The listing builds one solid part. Answer for the finished solid, in the listing's coordinates (mm). Coordinates: 2 decimals unless noted, no trailing zeros. Order: outer loops, then holes, each group sorted by start corner. A loop starts at its lowest first (then second) coordinate and runs counter-clockwise, first axis right, second up. Notation, with made-up numbers: (-22, 53.25) -> (19, 53.25) arc R12 ccw to (19, 57.25) -> close; hole circle Ø8 at (71, 16.25). An arc over 180 degrees is marked (long way). Answer in a Markdown table with one row per item. Add a question column.
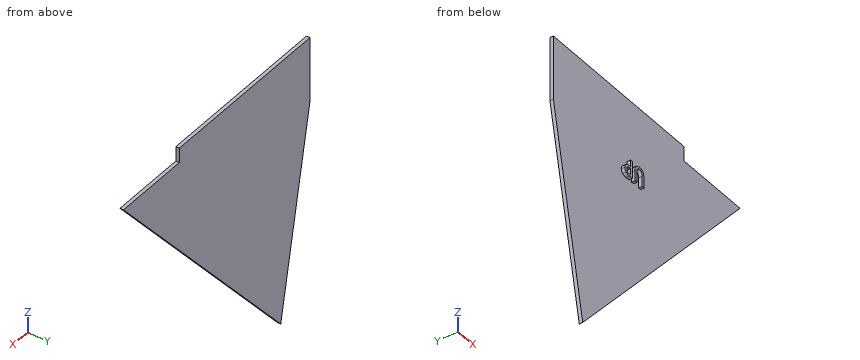
```python
from build123d import *

# Parameters (mm, degrees)
EXTRUDE_1_DEPTH = 1
EXTRUDE_2_DEPTH = 1


with BuildPart() as part:
    # 草图1 → 凸台-拉伸1 (new body)
    with BuildSketch(Plane(origin=(0, 0, 0), x_dir=(1, 0, 0), z_dir=(0, 1, 0))):
        Polygon((12.66597943, 73.92266442), (1, 15.376339461), (1, -3.25), (53, -3.25), (53, 1), (75.227111726, 1), align=None)
    extrude(amount=EXTRUDE_1_DEPTH)

    # 草图2 → 凸台-拉伸2 (add)
    # profile 1 of 2: a face of its own
    with BuildSketch(Plane(origin=(0, 0, 0), x_dir=(1, 0, 0), z_dir=(0, 1, 0))):
        with BuildLine():
            Line((31.090740008, 15.394221889), (30.323543176, 15.394221889))
            Line((30.323543176, 15.394221889), (30.323543176, 17.352620355))
            add(Edge.make_bspline(
                [(30.323543176, 17.352620355), (30.291480188, 17.346927632), (30.225432017, 17.335200902), (30.122464474, 17.325658206), (30.013401991, 17.319675849), (29.938694803, 17.319783871), (29.900262675, 17.319839442)],
                knots=[0, 0, 0, 0, 0.918585764, 1.892241272, 2.915691322, 4, 4, 4, 4], degree=3))
            add(Edge.make_bspline(
                [(29.900262675, 17.319839442), (29.841962947, 17.319869767), (29.726722993, 17.319929711), (29.556261285, 17.335932691), (29.390055361, 17.361937179), (29.228423578, 17.400915644), (29.070924954, 17.451283461), (28.917434146, 17.512464376), (28.768763104, 17.586671732), (28.62561681, 17.671704257), (28.490911455, 17.769835394), (28.373499458, 17.887220571), (28.271718538, 18.019975809), (28.188806413, 18.170044776), (28.12115622, 18.335792286), (28.072018776, 18.517995324), (28.038306105, 18.716089526), (28.030646768, 18.853776873), (28.026679563, 18.925092951)],
                knots=[0, 0, 0, 0, 1.003522523, 1.98364375, 2.944869411, 3.898614004, 4.843729631, 5.790462383, 6.741287792, 7.702146141, 8.655643954, 9.602935836, 10.551034771, 11.527201242, 12.5464735, 13.626777097, 14.770773406, 16, 16, 16, 16], degree=3))
            add(Edge.make_bspline(
                [(28.026679563, 18.925092951), (28.029126999, 18.981235603), (28.033891792, 19.09053695), (28.057781565, 19.249075834), (28.094861108, 19.397722477), (28.143989367, 19.537154386), (28.209760487, 19.66561534), (28.285926292, 19.785665607), (28.377011339, 19.895385017), (28.447566531, 19.958919299), (28.483028853, 19.990852784)],
                knots=[0, 0, 0, 0, 1.126595518, 2.193312949, 3.209115705, 4.196248007, 5.151139266, 6.097382339, 7.043709754, 8, 8, 8, 8], degree=3))
            add(Edge.make_bspline(
                [(28.483028853, 19.990852784), (28.522929015, 20.023049122), (28.603984669, 20.088454754), (28.741989665, 20.169383539), (28.893542525, 20.238034743), (29.059185588, 20.295093718), (29.239564674, 20.338290061), (29.434352813, 20.367230207), (29.64317297, 20.387190847), (29.787147929, 20.388758207), (29.861524951, 20.3895679)],
                knots=[0, 0, 0, 0, 0.838628006, 1.70364077, 2.610636308, 3.559859354, 4.568055018, 5.643200099, 6.782484425, 8, 8, 8, 8], degree=3))
            add(Edge.make_bspline(
                [(29.861524951, 20.3895679), (29.924201068, 20.388442465), (30.046421709, 20.386247828), (30.224716607, 20.380809359), (30.393254737, 20.372443419), (30.551968816, 20.360836156), (30.701043327, 20.348103258), (30.840301091, 20.33201309), (30.969478734, 20.313349379), (31.052038447, 20.298457491), (31.091683908, 20.291306355)],
                knots=[0, 0, 0, 0, 1.217605855, 2.374374404, 3.464660226, 4.494999595, 5.465333604, 6.370582827, 7.217548217, 8, 8, 8, 8], degree=3))
            Line((31.091683908, 20.291306355), (31.090740008, 15.394221889))
        make_face()
        with BuildLine():
            add(Edge.make_bspline(
                [(30.323543176, 19.750609507), (30.294001104, 19.756441871), (30.227115227, 19.76964686), (30.11276139, 19.781736761), (29.973146382, 19.790998313), (29.871306917, 19.79377259), (29.816173468, 19.795274517)],
                knots=[0, 0, 0, 0, 0.708180311, 1.603383121, 2.702528978, 4, 4, 4, 4], degree=3))
            add(Edge.make_bspline(
                [(29.816173468, 19.795274517), (29.778674753, 19.794489016), (29.705419893, 19.792954518), (29.598288212, 19.782736487), (29.496988537, 19.764581207), (29.401019543, 19.740409824), (29.311269908, 19.708215699), (29.227058284, 19.669148461), (29.148784868, 19.623070355), (29.076655109, 19.569835898), (29.010798742, 19.510512464), (28.953667436, 19.442775826), (28.905730333, 19.367849012), (28.86536387, 19.286573026), (28.83427513, 19.198006126), (28.811939273, 19.102330333), (28.797510474, 18.999843052), (28.79510899, 18.929236118), (28.793875472, 18.892968984)],
                knots=[0, 0, 0, 0, 1.164286524, 2.274468469, 3.33712435, 4.356941393, 5.343590938, 6.292901648, 7.23538906, 8.158502959, 9.072142365, 9.981112688, 10.900594105, 11.827687296, 12.792632354, 13.80775062, 14.873954761, 16, 16, 16, 16], degree=3))
            add(Edge.make_bspline(
                [(28.793875472, 18.892968984), (28.795134881, 18.854191832), (28.797580351, 18.778895935), (28.811554204, 18.669650618), (28.835574304, 18.567590725), (28.867328792, 18.472146789), (28.907923347, 18.383372416), (28.95859169, 18.302223365), (29.018603775, 18.228366562), (29.086740761, 18.16077878), (29.163691225, 18.101659974), (29.247154269, 18.048964292), (29.338736059, 18.005658508), (29.437186031, 17.969976467), (29.54264825, 17.941254338), (29.655625397, 17.922037488), (29.775583455, 17.909511306), (29.858027897, 17.907569166), (29.900262675, 17.906574244)],
                knots=[0, 0, 0, 0, 1.10647952, 2.148516939, 3.135813804, 4.093347323, 5.013956832, 5.913991464, 6.814877829, 7.723438285, 8.645449828, 9.577866136, 10.534345172, 11.529217628, 12.562346088, 13.648092354, 14.795160789, 16, 16, 16, 16], degree=3))
            add(Edge.make_bspline(
                [(29.900262675, 17.906574244), (29.941533493, 17.906028809), (30.020359402, 17.904987046), (30.132306289, 17.911998092), (30.23270458, 17.922996362), (30.294355499, 17.937500422), (30.323543176, 17.944367146)],
                knots=[0, 0, 0, 0, 1.161518353, 2.218461969, 3.156558288, 4, 4, 4, 4], degree=3))
            Line((30.323543176, 17.944367146), (30.323543176, 19.750609507))
        make_face(mode=Mode.SUBTRACT)
    # profile 2 of 2: a face of its own
    with BuildSketch(Plane(origin=(0, 0, 0), x_dir=(1, 0, 0), z_dir=(0, 1, 0))):
        with BuildLine():
            Line((32.077134748, 20.358527157), (32.844331579, 20.358527157))
            Line((32.844331579, 20.358527157), (32.844331579, 17.334805283))
            add(Edge.make_bspline(
                [(32.844331579, 17.334805283), (32.846041524, 17.274995945), (32.849340681, 17.159600138), (32.862116571, 16.992717533), (32.883577596, 16.838338831), (32.913517977, 16.696138778), (32.951987807, 16.566089797), (32.999008574, 16.448639235), (33.054117718, 16.34331339), (33.117299737, 16.250152646), (33.189122104, 16.169354435), (33.266600201, 16.098618835), (33.351533105, 16.040070587), (33.442049228, 15.99081552), (33.539783431, 15.954258392), (33.643837974, 15.928897808), (33.754040259, 15.91342912), (33.829727782, 15.911895168), (33.868517376, 15.911109023)],
                knots=[0, 0, 0, 0, 1.442558911, 2.783265207, 4.033293762, 5.19797452, 6.283894868, 7.299176403, 8.243481286, 9.144954945, 10.005756174, 10.844503658, 11.66816234, 12.486940923, 13.323278702, 14.176003432, 15.065208066, 16, 16, 16, 16], degree=3))
            add(Edge.make_bspline(
                [(33.868517376, 15.911109023), (33.904473646, 15.911526383), (33.97484436, 15.912343207), (34.077658287, 15.92781335), (34.174878032, 15.954543092), (34.267116792, 15.991646317), (34.354322253, 16.038718034), (34.435688698, 16.097382655), (34.511493017, 16.167040691), (34.582608735, 16.247198802), (34.646508679, 16.340053843), (34.701762221, 16.445170296), (34.749598601, 16.562786913), (34.787162737, 16.693178193), (34.818776759, 16.835728654), (34.84076289, 16.990817804), (34.855116558, 17.158326046), (34.857473172, 17.274141756), (34.858691406, 17.33401178)],
                knots=[0, 0, 0, 0, 0.880869997, 1.723967724, 2.54076827, 3.348096003, 4.15667844, 4.964596865, 5.80091263, 6.676282017, 7.586647838, 8.557371955, 9.582678263, 10.694376867, 11.880403812, 13.160330013, 14.532054847, 16, 16, 16, 16], degree=3))
            Line((34.858691406, 17.33401178), (34.858691406, 20.358527157))
            Line((34.858691406, 20.358527157), (35.625888237, 20.358527157))
            Line((35.625888237, 20.358527157), (35.625888237, 17.380520301))
            add(Edge.make_bspline(
                [(35.625888237, 17.380520301), (35.623936714, 17.291573771), (35.620165761, 17.119701207), (35.595302232, 16.872154063), (35.557140127, 16.644043754), (35.504575812, 16.435278366), (35.438009439, 16.245400882), (35.356778606, 16.074929633), (35.261228593, 15.923975043), (35.150246411, 15.793333485), (35.02731822, 15.680891375), (34.895571803, 15.582265655), (34.752268142, 15.501033739), (34.599951136, 15.43349429), (34.437335243, 15.382310688), (34.264956857, 15.348185822), (34.083249013, 15.326302213), (33.958656361, 15.325651598), (33.894972407, 15.325319044)],
                knots=[0, 0, 0, 0, 1.389947096, 2.68581329, 3.884176986, 5.001519278, 6.046082896, 7.023506491, 7.946473535, 8.830015835, 9.69383004, 10.545329235, 11.396344648, 12.262399475, 13.145009074, 14.054291982, 15.00547603, 16, 16, 16, 16], degree=3))
            add(Edge.make_bspline(
                [(33.894972407, 15.325319044), (33.828469528, 15.326101711), (33.698576147, 15.327630415), (33.508729563, 15.348474132), (33.329189291, 15.385576465), (33.159391405, 15.436827956), (33.000035358, 15.505949179), (32.850490052, 15.58964615), (32.711713219, 15.690227791), (32.581893571, 15.804556755), (32.464864256, 15.937598686), (32.363164513, 16.09050188), (32.277381449, 16.262754247), (32.206934074, 16.45360011), (32.151146625, 16.663013971), (32.111664078, 16.891642935), (32.084450881, 17.139060264), (32.080248305, 17.310628986), (32.078078648, 17.399204536)],
                knots=[0, 0, 0, 0, 1.013962662, 1.980471211, 2.907472823, 3.806985122, 4.680561309, 5.551651082, 6.415505808, 7.289926821, 8.185106327, 9.109702809, 10.082849364, 11.113391155, 12.207519227, 13.383461846, 14.649163417, 16, 16, 16, 16], degree=3))
            Line((32.078078648, 17.399204536), (32.077134748, 20.358527157))
        make_face()
    extrude(amount=-EXTRUDE_2_DEPTH)


solid = part.part
```
Q1. Straight lines are drawn through the part: line 1 (Y direction, x = 17, z = -53); line 2 (X direction, y = 0.9, z = -29); line 3 (X direction, y = 0.55, z = -15.5). For each, find the intervals that lie inside material, in ascending order.
Q2. Given pin 1 (0.8 mm diameter, centred on y = -0.5, z = -16.5, fed in from +X); pin 2 (0.8 mm diameter, centred on x = 64.5, y = 0.5, fed in from +Z); pin 3 (0.8 mm diameter, centred on y = -0.5, z = -19, fed in from -X), each flat-ended and moving along its own axis, determine where each tip first touches the part or whether it passes through.
Q3. A cutting plane is placed at A-A (y = -0.6). State how many separate pieces and enclosed holes the cut face has, then the cut area to 3 significant figures.
Q4. A cutting plane is placed at B-B (x = 49). Determine the outline of the cut face in (y, z).
Q5. A cutting plane is placed at C-C (z = -43.5). Determine the outline of the cut face in (x, y).
Returned:
| question | item | result |
|---|---|---|
| 1 | line 1 | y = 0 to 1 |
| 1 | line 2 | x = 3.71 to 51.21 |
| 1 | line 3 | x = 1.02 to 62.79 |
| 2 | pin 1 | stops at x = 35.6 |
| 2 | pin 2 | stops at z = -1 |
| 2 | pin 3 | stops at x = 28.03 |
| 3 | separate pieces | 2 |
| 3 | enclosed holes | 1 |
| 3 | area | 15.4 mm² |
| 4 | outline | (0, -31.57) -> (1, -31.57) -> (1, 3.25) -> (0, 3.25) -> close |
| 5 | outline | (6.6, 0) -> (38.77, 0) -> (38.77, 1) -> (6.6, 1) -> close |
